Work out the finished part from the listing and answer in its coordinate system (mm). Round coordinates to 2 decimals unless told otherwise and drop trailing zeros. Order: outer loops, then holes, each group sorted by start corner. A loop starts at its lowest first (then second) coordinate and runs counter-clockwise, first axis right, second up. Notation, with made-up numbers: (24, -34) -> (59, -34) arc R28 cw to (59, -6) -> close; hole circle Ø6 at (12.25, 27.5). An arc over 180 degrees is marked (long way). Use one line per item in the form item = value.
```python
from build123d import *

# Parameters (mm, degrees)
SKETCH1_W             = 73.66
SKETCH1_H             = 141.478
PLATE_DEPTH           = 3.175
SKETCH2_W             = 73.66
SKETCH2_H             = 141.478
SKETCH2_W_2           = 68.58
SKETCH2_H_2           = 136.398
WALLS_DEPTH           = 10.576866729
LIP_W                 = 87.63
LIP_H                 = 147.828
LIP_W_2               = 73.66
LIP_H_2               = 141.478
FLANGE_DEPTH          = 2.54
FILLET1_R             = 12.7
FILLET2_R             = 3.175
FILLET3_R             = 1.27
SKETCH16_W            = 5.715
SKETCH16_H            = 6.35
EXTRUDE4_DEPTH        = 7.401866729
FILLET6_R             = 3.175
F_6_CLEARANCE_HOLE1_D = 3.7973
F_1_64_TAPPED_HOLE1_D = 1.8542
CUT_EXTRUDE7_DEPTH    = 87.573112055
FILLET7_R             = 1.5875
FILLET7_OF_MIRROR5_R  = 1.5875
MIRROR6_DEPTH         = 3.175
F_4_CLEAR_MID_D       = 3.4544
HOLE_PAT_COUNT        = 3
HOLE_PAT_PITCH        = 15.875
HOLE_PAT_COL_COUNT    = 2
HOLE_PAT_COL_PITCH    = 15.875
MIRROR7_COPY_1_D      = 3.4544
MIRROR7_COPY_2_D      = 3.4544
MIRROR7_COPY_3_D      = 3.4544
MIRROR7_COPY_4_D      = 3.4544


# Read off the part's stored shape, not the designer's step: Mirror6
with BuildPart() as part:
    # Sketch1 → plate (new body)
    with BuildSketch(Plane.XY):
        Rectangle(SKETCH1_W, SKETCH1_H)
    extrude(amount=PLATE_DEPTH)

    # Sketch2 → walls (add)
    with BuildSketch(Plane.XY):
        Rectangle(SKETCH2_W, SKETCH2_H)
        Rectangle(SKETCH2_W_2, SKETCH2_H_2, mode=Mode.SUBTRACT)
    extrude(amount=WALLS_DEPTH)

    # lip → flange (add)
    with BuildSketch(Plane(origin=(0, 0, 6.131866729), x_dir=(1, 0, 0), z_dir=(0, 0, -1))):
        Rectangle(LIP_W, LIP_H)
        Rectangle(LIP_W_2, LIP_H_2, mode=Mode.SUBTRACT)
    extrude(amount=FLANGE_DEPTH)

    # Fillet1
    fillet1_edges = [part.edges().sort_by_distance(p)[0] for p in [
        (-43.815, 73.914, 4.861866729),
        (43.815, 73.914, 4.861866729),
        (43.815, -73.914, 4.861866729),
        (-43.815, -73.914, 4.861866729),
    ]]
    fillet(fillet1_edges, radius=FILLET1_R)

    # Fillet2
    fillet2_edges = [part.edges().sort_by_distance(p)[0] for p in [
        (34.29, -68.199, 6.875933364),
        (34.29, 68.199, 6.875933364),
        (-34.29, 68.199, 6.875933364),
        (-34.29, -68.199, 6.875933364),
        (-36.83, -70.739, 1.795933365),
        (-36.83, 70.739, 1.795933365),
        (36.83, 70.739, 1.795933365),
        (36.83, -70.739, 1.795933365),
        (-36.83, -70.739, 8.354366729),
        (-36.83, 70.739, 8.354366729),
        (36.83, 70.739, 8.354366729),
        (36.83, -70.739, 8.354366729),
    ]]
    fillet(fillet2_edges, radius=FILLET2_R)

    # Fillet3
    fillet3_edges = [part.edges().sort_by_distance(p)[0] for p in [
        (0, 70.739, 10.576866729),
        (0, -70.739, 10.576866729),
        (36.83, 0, 10.576866729),
        (-35.90006403, -69.80906403, 10.576866729),
        (35.90006403, -69.80906403, 10.576866729),
        (35.90006403, 69.80906403, 10.576866729),
        (-35.90006403, 69.80906403, 10.576866729),
        (-36.83, 0, 10.576866729),
    ]]
    fillet(fillet3_edges, radius=FILLET3_R)

    # Sketch16 → Extrude4 (add)
    with BuildSketch(Plane.XY.offset(3.175)):
        with Locations((-31.4325, 0)):
            Rectangle(SKETCH16_W, SKETCH16_H)
    extrude4 = extrude(amount=EXTRUDE4_DEPTH)

    # Sketch12 → #6-32 Tapped Hole1 (revolve, cut)
    with BuildSketch(Plane(origin=(-31.4325, 0, 10.576866729), x_dir=(0, -1, 0), z_dir=(1, 0, 0))):
        Polygon((0, 0), (0, 10.20053403), (1.35255, 9.38784), (1.35255, 7.0104), (1.7526, 7.0104), (1.7526, 0), align=None)
    f_6_32_tapped_hole1 = revolve(axis=Axis((-31.4325, 0, 16.926866729), (0, 0, -1)), mode=Mode.SUBTRACT)

    # Mirror4: Extrude4, #6-32 Tapped Hole1 across plane
    add(extrude4.mirror(Plane(origin=(0, 0, 0), x_dir=(0, 0, 1), z_dir=(1, 0, 0))))
    add(f_6_32_tapped_hole1.mirror(Plane(origin=(0, 0, 0), x_dir=(0, 0, 1), z_dir=(1, 0, 0))), mode=Mode.SUBTRACT)

    # Fillet6
    fillet6_edges = [part.edges().sort_by_distance(p)[0] for p in [
        (-34.29, -3.175, 6.875933364),
        (-34.29, 3.175, 6.875933364),
        (34.29, -3.175, 6.875933364),
        (34.29, 3.175, 6.875933364),
    ]]
    fillet(fillet6_edges, radius=FILLET6_R)

    # #6 Clearance Hole1 (through all)
    with Locations(Plane(origin=(-40.3225, -57.15, 6.131866729), x_dir=(0, 1, 0), z_dir=(0, 0, 1))):
        with Locations((0, 0), (38.1, 0), (114.3, 0), (76.2, 0)):
            f_6_clearance_hole1 = Hole(F_6_CLEARANCE_HOLE1_D / 2)

    # #1-64 Tapped Hole1 (through all)
    with Locations(Plane(origin=(-40.3225, -38.1, 6.131866729), x_dir=(0, 1, 0), z_dir=(0, 0, 1))):
        with Locations((0, 0), (76.2, 0)):
            f_1_64_tapped_hole1 = Hole(F_1_64_TAPPED_HOLE1_D / 2)

    # Mirror3: #6 Clearance Hole1, #1-64 Tapped Hole1 across plane
    add(f_6_clearance_hole1.mirror(Plane(origin=(0, 0, 0), x_dir=(0, 0, 1), z_dir=(1, 0, 0))), mode=Mode.SUBTRACT)
    add(f_1_64_tapped_hole1.mirror(Plane(origin=(0, 0, 0), x_dir=(0, 0, 1), z_dir=(1, 0, 0))), mode=Mode.SUBTRACT)

    # cutout → Cut-Extrude7 (cut, through all)
    with BuildSketch(Plane.XY):
        Polygon((0, 0), (0, 62.2173), (-32.385, 62.2173), (-32.385, 9.525), (-28.575, 9.525), (-28.575, 0), align=None)
    cut_extrude7 = extrude(amount=CUT_EXTRUDE7_DEPTH, mode=Mode.SUBTRACT)

    # Fillet7
    fillet7_edges = [part.edges().sort_by_distance(p)[0] for p in [
        (-32.385, 62.2173, 1.5875),
        (-32.385, 9.525, 1.5875),
    ]]
    fillet(fillet7_edges, radius=FILLET7_R)

    # Mirror5: Cut-Extrude7 across plane
    add(cut_extrude7.mirror(Plane.ZX), mode=Mode.SUBTRACT)

    # Fillet7 of Mirror5
    fillet7_of_mirror5_edges = [part.edges().sort_by_distance(p)[0] for p in [
        (-32.385, -62.2173, 1.5875),
        (-32.385, -9.525, 1.5875),
    ]]
    fillet(fillet7_of_mirror5_edges, radius=FILLET7_OF_MIRROR5_R)

    # Mirror6 outline → Mirror6 (cut)
    with BuildSketch(Plane.XY):
        with BuildLine():
            Line((28.575, -9.525), (28.575, 9.525))
            Line((28.575, 9.525), (30.7975, 9.525))
            ThreePointArc((30.7975, 9.525), (31.920032015, 9.989967985), (32.385, 11.1125))
            Line((32.385, 11.1125), (32.385, 60.6298))
            ThreePointArc((32.385, 60.6298), (31.920032015, 61.752332015), (30.7975, 62.2173))
            Line((30.7975, 62.2173), (0, 62.2173))
            Line((0, 62.2173), (0, -62.2173))
            Line((0, -62.2173), (30.7975, -62.2173))
            ThreePointArc((30.7975, -62.2173), (31.920032015, -61.752332015), (32.385, -60.6298))
            Line((32.385, -60.6298), (32.385, -11.1125))
            ThreePointArc((32.385, -11.1125), (31.920032015, -9.989967985), (30.7975, -9.525))
            Line((30.7975, -9.525), (28.575, -9.525))
        make_face()
    extrude(amount=MIRROR6_DEPTH, mode=Mode.SUBTRACT)

    # #4 Clear Mid (through all)
    with Locations(Plane.XY.offset(3.175)):
        with Locations((-7.9375, 65.20815)):
            f_4_clear_mid = Hole(F_4_CLEAR_MID_D / 2)

    # hole pat: #4 Clear Mid ×3
    with Locations(*[(i * HOLE_PAT_PITCH, 0, 0) for i in range(1, HOLE_PAT_COUNT)]):
        add(f_4_clear_mid, mode=Mode.SUBTRACT)

    # hole pat col: #4 Clear Mid ×2
    with Locations(*[(-i * HOLE_PAT_COL_PITCH, 0, 0) for i in range(1, HOLE_PAT_COL_COUNT)]):
        add(f_4_clear_mid, mode=Mode.SUBTRACT)

    # Mirror7 copy 1 (through all)
    with Locations(Plane(origin=(15.875, 0, 3.175), x_dir=(1, 0, 0), z_dir=(0, 0, 1))):
        with Locations((-7.9375, -65.20815)):
            Hole(MIRROR7_COPY_1_D / 2)

    # Mirror7 copy 2 (through all)
    with Locations(Plane(origin=(31.75, 0, 3.175), x_dir=(1, 0, 0), z_dir=(0, 0, 1))):
        with Locations((-7.9375, -65.20815)):
            Hole(MIRROR7_COPY_2_D / 2)

    # Mirror7 copy 3 (through all)
    with Locations(Plane(origin=(-15.875, 0, 3.175), x_dir=(1, 0, 0), z_dir=(0, 0, 1))):
        with Locations((-7.9375, -65.20815)):
            Hole(MIRROR7_COPY_3_D / 2)

    # Mirror7 copy 4 (through all)
    with Locations(Plane.XY.offset(3.175)):
        with Locations((-7.9375, -65.20815)):
            Hole(MIRROR7_COPY_4_D / 2)


solid = part.part
```
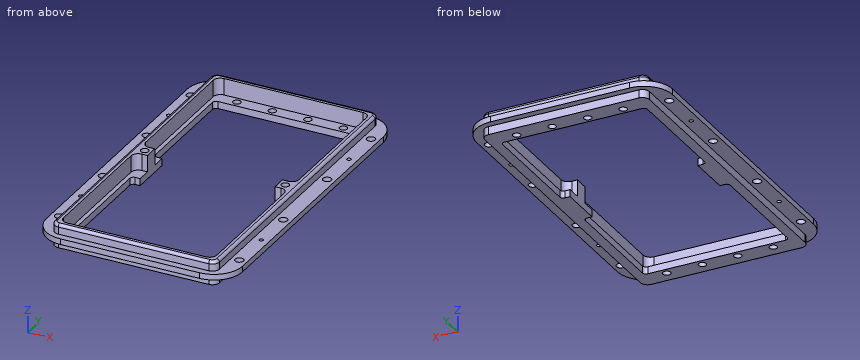
Item 1: Flat-ended cylindrical pins translate along their axes: P1, Ø2, axis at x = 30.5, z = 7.5, coming from the -Y side; P2, Ø2.5, axis at y = -12.5, z = 7.5, coming from the +X side; P3, Ø2.5, axis at x = 40.32, y = -38.1, coming from the +Z side; P4, Ø5, axis at y = -42.5, z = 3.5, coming from the +X side (3 decimals). Find the tip coordinate at first contact, or state that the pin passes through.
Findings:
P1 = -70.74
P2 = 36.83
P3 = 6.13
P4 = 43.815
Item 2: The part is cut by section B-B, the plane y = -49.5. Give the vertices of the cut face in (x, z) (3 decimals).
Findings:
outline = (-43.815, 3.592) -> (-36.83, 3.592) -> (-36.83, 0) -> (-32.385, 0) -> (-32.385, 3.175) -> (-34.29, 3.175) -> (-34.29, 10.577) -> (-35.56, 10.577) arc R1.27 ccw to (-36.83, 9.307) -> (-36.83, 6.132) -> (-43.815, 6.132) -> close; (32.385, 0) -> (36.83, 0) -> (36.83, 3.592) -> (43.815, 3.592) -> (43.815, 6.132) -> (36.83, 6.132) -> (36.83, 9.307) arc R1.27 ccw to (35.56, 10.577) -> (34.29, 10.577) -> (34.29, 3.175) -> (32.385, 3.175) -> close
Item 3: Consider line 1 along X through (y, z) = (-57.15, 4.7) (3 decimals); line 2 along Y through (x, z) = (31.5, 9.5); line 3 along Y through (x, z) = (-5.5, 0.75). Determine where each line is inside the solid, lowest interval first.
Findings:
line_1 = -43.815 to -42.221, -38.424 to -34.29, 34.29 to 38.424, 42.221 to 43.815
line_2 = -70.72 to -68.18, -3.2 to -1.75, 1.75 to 3.2, 68.18 to 70.72
line_3 = -70.74 to -62.22, 62.22 to 70.74
Item 4: The part is cut by section C-C, the plane y = 57.15. Give the number of separate pieces and of enclosed holes in the cut face, and give its area (3 significant figures).
Findings:
separate_pieces = 4
enclosed_holes = 0
area = 81.3 mm^2
Item 5: The part is cut by section A-A, the plane x = -12.5. Give the vertices of the cut face in (y, z) (3 decimals).
Findings:
outline = (-73.914, 3.592) -> (-70.739, 3.592) -> (-70.739, 0) -> (-62.217, 0) -> (-62.217, 3.175) -> (-68.199, 3.175) -> (-68.199, 10.577) -> (-69.469, 10.577) arc R1.27 ccw to (-70.739, 9.307) -> (-70.739, 6.132) -> (-73.914, 6.132) -> close; (62.217, 0) -> (70.739, 0) -> (70.739, 3.592) -> (73.914, 3.592) -> (73.914, 6.132) -> (70.739, 6.132) -> (70.739, 9.307) arc R1.27 ccw to (69.469, 10.577) -> (68.199, 10.577) -> (68.199, 3.175) -> (62.217, 3.175) -> close
